Autodesk Inventor part; units mm, degrees
ref_plane "YZ Plane" through (0, 0, 0) normal (1, 0, 0) x (0, 1, 0)
ref_plane "XZ Plane" through (0, 0, 0) normal (0, 1, 0) x (-1, 0, 0)
ref_plane "XY Plane" through (0, 0, 0) normal (0, 0, 1) x (1, 0, 0)
sketch "Sketch1" plane through (0, 0, 0) normal (0, 0, 1) x (1, 0, 0)
  line L0 (-34.86, 0) -> (34.86, 0) construction
  line L1 (0, -34.86) -> (0, 34.86) construction
  line L2 (0, 0) -> (11.157509, 11.157509) construction
  line L3 (0, 0) -> (15.7791, 0) construction
  line L4 (0, 24.9) -> (16.800857, 24.9)
  line L5 (16.800857, 24.9) -> (16.800857, 21.241488)
  line L6 (16.800857, 21.241488) -> (19.021172, 19.021172)
  line L7 (24.9, 0) -> (24.9, 16.800857)
  line L8 (24.9, 16.800857) -> (21.241488, 16.800857)
  line L9 (21.241488, 16.800857) -> (19.021172, 19.021172)
  line L10 (0, -24.9) -> (16.800857, -24.9)
  line L11 (16.800857, -24.9) -> (16.800857, -21.241488)
  line L12 (16.800857, -21.241488) -> (19.021172, -19.021172)
  line L13 (24.9, 0) -> (24.9, -16.800857)
  line L14 (24.9, -16.800857) -> (21.241488, -16.800857)
  line L15 (21.241488, -16.800857) -> (19.021172, -19.021172)
  line L16 (0, 24.9) -> (-16.800857, 24.9)
  line L17 (-16.800857, 24.9) -> (-16.800857, 21.241488)
  line L18 (-16.800857, 21.241488) -> (-19.021172, 19.021172)
  line L19 (-24.9, 16.800857) -> (-21.241488, 16.800857)
  line L20 (-21.241488, 16.800857) -> (-19.021172, 19.021172)
  line L21 (0, -24.9) -> (-16.800857, -24.9)
  line L22 (-16.800857, -24.9) -> (-16.800857, -21.241488)
  line L23 (-16.800857, -21.241488) -> (-19.021172, -19.021172)
  line L24 (-21.241488, -16.800857) -> (-19.021172, -19.021172)
  line L25 (-24.9, -16.800857) -> (-21.241488, -16.800857)
  line L26 (-24.9, 0) -> (-24.9, -16.800857)
  line L27 (-24.9, 0) -> (-24.9, 16.800857)
  circle A0 centre (0, 0) radius 12.5
  dimension "d0" = 45
  dimension "d2" = 24.9
  dimension "d3" = 3.14
  dimension "d4" = 26.9
  dimension "d5" = 25
extrude "Extrusion1" add sketch "Sketch1" along normal blind 6
sketch "Sketch4" plane through (0, 0, 0) normal (0, 0, -1) x (-1, 0, 0)
  circle A0 centre (0, 0) radius 12.5 construction
  line L0 (16.800857, 24.9) -> (-16.800857, 24.9) construction
  line L1 (-16.800857, 24.9) -> (-16.800857, 21.241488)
  line L2 (-16.800857, 21.241488) -> (-21.241488, 16.800857)
  line L3 (-21.241488, 16.800857) -> (-24.9, 16.800857)
  line L4 (-24.9, 16.800857) -> (-24.9, -16.800857) construction
  line L5 (-24.9, -16.800857) -> (-21.241488, -16.800857)
  line L6 (-21.241488, -16.800857) -> (-16.800857, -21.241488)
  line L7 (-16.800857, -21.241488) -> (-16.800857, -24.9)
  line L8 (-16.800857, -24.9) -> (16.800857, -24.9) construction
  line L9 (16.800857, -24.9) -> (16.800857, -21.241488)
  line L10 (16.800857, -21.241488) -> (21.241488, -16.800857)
  line L11 (21.241488, -16.800857) -> (24.9, -16.800857)
  line L12 (24.9, -16.800857) -> (24.9, 16.800857) construction
  line L13 (24.9, 16.800857) -> (21.241488, 16.800857)
  line L14 (21.241488, 16.800857) -> (16.800857, 21.241488)
  line L15 (16.800857, 21.241488) -> (16.800857, 24.9)
  line L16 (-17.000857, 25.1) -> (17.000857, 25.1) construction
  line L17 (17.000857, 25.1) -> (17.000857, 21.32433)
  line L18 (17.000857, 21.32433) -> (21.32433, 17.000857)
  line L19 (21.32433, 17.000857) -> (25.1, 17.000857)
  line L20 (25.1, 17.000857) -> (25.1, -17.000857) construction
  line L21 (25.1, -17.000857) -> (21.32433, -17.000857)
  line L22 (21.32433, -17.000857) -> (17.000857, -21.32433)
  line L23 (17.000857, -21.32433) -> (17.000857, -25.1)
  line L24 (17.000857, -25.1) -> (-17.000857, -25.1) construction
  line L25 (-17.000857, -25.1) -> (-17.000857, -21.32433)
  line L26 (-17.000857, -21.32433) -> (-21.32433, -17.000857)
  line L27 (-21.32433, -17.000857) -> (-25.1, -17.000857)
  line L28 (-25.1, -17.000857) -> (-25.1, 17.000857) construction
  line L29 (-25.1, 17.000857) -> (-21.32433, 17.000857)
  line L30 (-21.32433, 17.000857) -> (-17.000857, 21.32433)
  line L31 (-17.000857, 21.32433) -> (-17.000857, 25.1)
  line L32 (-24.9, -16.800857) -> (-24.9, 16.800857)
  line L33 (-24.9, 16.800857) -> (-24.9, 17.000857)
  line L34 (-16.800857, 24.9) -> (-17.000857, 24.9)
  line L35 (-16.800857, 24.9) -> (16.800857, 24.9)
  line L36 (16.800857, 24.9) -> (17.000857, 24.9)
  line L37 (24.9, 16.800857) -> (24.9, 17.000857)
  line L38 (24.9, 16.800857) -> (24.9, -16.800857)
  line L39 (24.9, -16.800857) -> (24.9, -17.000857)
  line L40 (16.800857, -24.9) -> (-16.800857, -24.9)
  line L41 (16.800857, -24.9) -> (17.000857, -24.9)
  line L42 (-16.800857, -24.9) -> (-17.000857, -24.9)
  line L43 (-24.9, -16.800857) -> (-24.9, -17.000857)
  dimension "d19" = 0.2
extrude "IM_offset" add sketch "Sketch4" against normal up to surface (6 mm away) contours L1 L2 L3 L33 L29 L30 L31 L34 | L36 L17 L18 L19 L37 L13 L14 L15 | L5 L6 L7 L42 L25 L26 L27 L43 | L39 L21 L22 L23 L41 L9 L10 L11
sketch "Skizze5" plane through (0, 0, 6) normal (0, 0, 1) x (1, 0, 0)
  circle A0 centre (0, 0) radius 12.5
  line L0 (-17.000857, 24.9) -> (17.000857, 24.9)
  line L1 (-17.000857, 21.32433) -> (-17.000857, 24.9)
  line L2 (-21.32433, 17.000857) -> (-17.000857, 21.32433)
  line L3 (-24.9, 17.000857) -> (-21.32433, 17.000857)
  line L4 (-24.9, -17.000857) -> (-24.9, 17.000857)
  line L5 (-21.32433, -17.000857) -> (-24.9, -17.000857)
  line L6 (-17.000857, -21.32433) -> (-21.32433, -17.000857)
  line L7 (-17.000857, -24.9) -> (-17.000857, -21.32433)
  line L8 (17.000857, -24.9) -> (-17.000857, -24.9)
  line L9 (17.000857, -21.32433) -> (17.000857, -24.9)
  line L10 (21.32433, -17.000857) -> (17.000857, -21.32433)
  line L11 (24.9, -17.000857) -> (21.32433, -17.000857)
  line L12 (24.9, 17.000857) -> (24.9, -17.000857)
  line L13 (21.32433, 17.000857) -> (24.9, 17.000857)
  line L14 (17.000857, 21.32433) -> (21.32433, 17.000857)
  line L15 (17.000857, 24.9) -> (17.000857, 21.32433)
  circle A1 centre (0, 0) radius 20
  circle A2 centre (0, 20) radius 4.05
  circle A3 centre (0, -20) radius 4.05
  dimension "d22" = 40
  dimension "d23" = 8.1
  dimension "d24" = 8.1
sketch "Skizze5 outline for Extrusion4" plane through (0, 0, 6) normal (0, 0, 1) x (1, 0, 0)
  circle A0 centre (0, -20) radius 4.05
  circle A1 centre (0, 20) radius 4.05
extrude "Extrusion4" cut sketch "Skizze5 outline for Extrusion4" against normal blind 5 draft -1
properties part number "20_Cube_insert_Sample_holder_v3"
Source: CAD feature listing. Evaluate the final solid. Frame: model axes, mm. A direction names the side the tool comes from. Coordinates: 2 decimals unless noted, no trailing zeros. Order: outer loops, then holes, each group sorted by start corner. A loop starts at its lowest first (then second) coordinate and runs counter-clockwise, first axis right, second up. Notation, with made-up numbers: M -35,-10.5 L -2,-10.5 A12 cw -2,6.5 Z; hole C 56,0.5 d8. An arc over 180 degrees is marked long. Write each question's results on one line, items separated by ' | '. Start each with the question number.
1. Draft query along Y for faces 4 (the face through (-17.001, -23, 3)), 5 (the face through (19.193, 19.132, 2.958)), 6 (the face through (0, 20, 1)). Return one class per face: +Y half, -Y half, draft (parallel to the pull), parting line (faces both ways), or undercut.
2. Section A-A, the plane y = -2.5. Return the cut outline in (x, z), then the cut area to 3 significant figures.
3. Material intervals for L1, parallel to Y at x = 0, z = 1.45; L2, parallel to Y at x = 0.5, z = 1.45; L3, parallel to X at y = -22, z = 0.65, sorted ascending.
4. Pin query (flat end, axial travel): pin 1 (1.1 mm diameter, centred on x = -22.5, z = 4, fed in from -Y); pin 2 (8 mm diameter, centred on x = -6.5, y = -7, fed in from -Z); pin 3 (3 mm diameter, centred on x = -24, z = 4, fed in from +Y); pin 4 (1.1 mm diameter, centred on y = -23.5, z = 2, fed in from +X). Return the tip coordinate at first contact, or that it passes through.
5. Reachability of faces 1 (the face through (17.001, -23, 3)), 2 (the face through (23, 17.001, 3)), 3 (the face through (-0.87, -23.91, 3.54)) from +Z, -Z, +X, -X, +Y, -Y: full face, straight path, thin tool, end or side. Return the list, or none.
6. Section B-B, the plane z = 3.85. Return the cut outline in (x, y), then the cut area to 3 significant figures.
7. Section C-C, the plane x = -19.5. Return the cut outline in (y, z).
Solution:
1) face 4: draft | face 5: +Y half | face 6: undercut
2) outline: M -24.9,0 L -12.25,0 L -12.25,6 L -24.9,6 Z; M 12.25,0 L 24.9,0 L 24.9,6 L 12.25,6 Z | area: 152 mm²
3) L1: -24.9 to -23.97, -16.03 to -12.5, 12.5 to 16.03, 23.97 to 24.9 | L2: -24.9 to -23.94, -16.06 to -12.49, 12.49 to 16.06, 23.94 to 24.9 | L3: -17 to 17
4) pin 1: y = -17 | pin 2: z = 0 | pin 3: y = 17 | pin 4: x = 17
5) face 1: +Z, -Z, +X, -Y | face 2: +Z, -Z, +X, +Y | face 3: +Z
6) outline: M -24.9,-17 L -21.32,-17 L -17,-21.32 L -17,-24.9 L 17,-24.9 L 17,-21.32 L 21.32,-17 L 24.9,-17 L 24.9,17 L 21.32,17 L 17,21.32 L 17,24.9 L -17,24.9 L -17,21.32 L -21.32,17 L -24.9,17 Z; hole C 0,0 d25; hole C 0,-20 d8.02; hole C 0,20 d8.02 | area: 1,680 mm²
7) outline: M -18.83,0 L 18.83,0 L 18.83,6 L -18.83,6 Z
